Autodesk Inventor part; units mm, degrees
ref_plane "YZ Plane" through (0, 0, 0) normal (1, 0, 0) x (0, 1, 0)
ref_plane "XZ Plane" through (0, 0, 0) normal (0, 1, 0) x (-1, 0, 0)
ref_plane "XY Plane" through (0, 0, 0) normal (0, 0, 1) x (1, 0, 0)
sketch "Sketch1" plane through (0, 0, 0) normal (0, 1, 0) x (-1, 0, 0)
  point P0 (0, 0)
sketch "Sketch2" plane through (0, 0, 0) normal (0, 1, 0) x (-1, 0, 0)
  line L0 (0, 0) -> (50.8, 0)
  line L1 (50.8, 0) -> (50.8, -50.8)
  line L2 (50.8, -50.8) -> (0, -50.8)
  line L3 (0, -50.8) -> (0, 0)
  line L4 (47.625, -47.625) -> (47.625, -3.175)
  line L5 (47.625, -3.175) -> (3.175, -3.175)
  line L6 (3.175, -3.175) -> (3.175, -47.625)
  line L7 (3.175, -47.625) -> (47.625, -47.625)
  line L8 (3.175, -3.175) -> (0, -3.175)
  line L9 (47.625, -47.625) -> (47.625, -50.8)
  dimension "d0" = 50.8
  dimension "d1" = 50.8
  dimension "d2" = 3.175
extrude "Extrusion1" add sketch "Sketch2" along normal blind 50.8 contours L0 L1 L2 L9 L4 L5 L8 L3
properties part number "AluminumBracket" material "Aluminum 6061"
Verification items for the finished model (mm, model axes). A direction names the side the tool comes from. Coordinates: 2 decimals unless noted, no trailing zeros. Order: outer loops, then holes, each group sorted by start corner. A loop starts at its lowest first (then second) coordinate and runs counter-clockwise, first axis right, second up. Notation, with made-up numbers: (24.25, 58.5) - (36.25, 58.5) arc R21 ccw to (36.25, 76.5) - close; hole circle Ø5 at (66.25, -30.75). An arc over 180 degrees is marked (long way). Return JSON: item names as keys, results as strings.
(1) Section check B-B, the plane x = -46.5. Record the cut outline in (y, z) (3 decimals).
Filled sheet:
{"outline": "(0, -3.175) - (50.8, -3.175) - (50.8, 0) - (0, 0) - close"}
(2) Thickness scan on line 1 along Z through (x, y) = (-11.5, 44) (3 decimals); line 2 along X through (y, z) = (34, -36.5) (3 decimals). Record the ranges inside material, lowest first.
Filled sheet:
{"line 1": "z = -3.175 to 0", "line 2": "x = -50.8 to -47.625"}
(3) Section check A-A, the plane y = 16. Record the cut outline in (x, z) (3 decimals), and give its area (4 significant figures).
Filled sheet:
{"outline": "(-50.8, -50.8) - (-47.625, -50.8) - (-47.625, -3.175) - (0, -3.175) - (0, 0) - (-50.8, 0) - close", "area": "312.5 mm^2"}
(4) Go/stop test with flat-tipped pins: pin 1 (3 mm diameter, centred on x = -12, y = 9.5, fed in from -Z) (3 decimals); pin 2 (5 mm diameter, centred on y = 44.5, z = -17, fed in from +X) (3 decimals). Record where each tip stops, or that it passes through.
Filled sheet:
{"pin 1": "stops at z = -3.175", "pin 2": "stops at x = -47.625"}
(5) Section check C-C, the plane z = -24.5. Record the cut outline in (x, y) (3 decimals), and give its area (3 significant figures).
Filled sheet:
{"outline": "(-50.8, 0) - (-47.625, 0) - (-47.625, 50.8) - (-50.8, 50.8) - close", "area": "161 mm^2"}
(6) Access from +Z, -Z, +X, -X, +Y, -Y to the whole of each face (thin tool, end or side, straight path). Record for faces 1 (the flat face through (0, 25, -2)), 2 (the flat face through (-24, 25, -3.175)).
Filled sheet:
{"face 1": "+Z, -Z, +X, +Y, -Y", "face 2": "-Z, +X, +Y, -Y"}
